from build123d import *

# Parameters (mm, degrees)
SKETCH1_R           = 16.995
SKETCH1_R_2         = 1.5
BOSS_EXTRUDE1_DEPTH = 5.08
CUT_EXTRUDE2_DEPTH  = 10


with BuildPart() as part:
    # Sketch1 → Boss-Extrude1 (new body)
    with BuildSketch(Plane.XY):
        Circle(SKETCH1_R)
        with Locations((-6.5, -11.258330249)):
            Circle(SKETCH1_R_2, mode=Mode.SUBTRACT)
        with Locations((6.5, -11.258330249)):
            Circle(SKETCH1_R_2, mode=Mode.SUBTRACT)
        with Locations((13, 0)):
            Circle(SKETCH1_R_2, mode=Mode.SUBTRACT)
        with Locations((6.5, 11.258330249)):
            Circle(SKETCH1_R_2, mode=Mode.SUBTRACT)
        with Locations((-6.5, 11.258330249)):
            Circle(SKETCH1_R_2, mode=Mode.SUBTRACT)
        with Locations((-13, 0)):
            Circle(SKETCH1_R_2, mode=Mode.SUBTRACT)
        with Locations((6.5, 11.258330249)):
            Circle(SKETCH1_R_2)
        with Locations((-6.5, -11.258330249)):
            Circle(SKETCH1_R_2)
    extrude(amount=BOSS_EXTRUDE1_DEPTH)

    # Sketch2 → Cut-Extrude2 (cut)
    with BuildSketch(Plane.XY.offset(5.08)):
        with BuildLine():
            ThreePointArc((-5.303300859, -8.131727984), (-5.303300859, -5.303300859), (-8.131727984, -5.303300859))
            Line((-8.131727984, -5.303300859), (-10.606601718, -7.778174593))
            ThreePointArc((-10.606601718, -7.778174593), (-10.606601718, -10.606601718), (-7.778174593, -10.606601718))
            Line((-7.778174593, -10.606601718), (-5.303300859, -8.131727984))
        make_face()
        with BuildLine():
            ThreePointArc((10.606601718, 7.778174593), (10.606601718, 10.606601718), (7.778174593, 10.606601718))
            Line((7.778174593, 10.606601718), (5.303300859, 8.131727984))
            ThreePointArc((5.303300859, 8.131727984), (5.303300859, 5.303300859), (8.131727984, 5.303300859))
            Line((8.131727984, 5.303300859), (10.606601718, 7.778174593))
        make_face()
    extrude(amount=-CUT_EXTRUDE2_DEPTH, mode=Mode.SUBTRACT)


solid = part.part
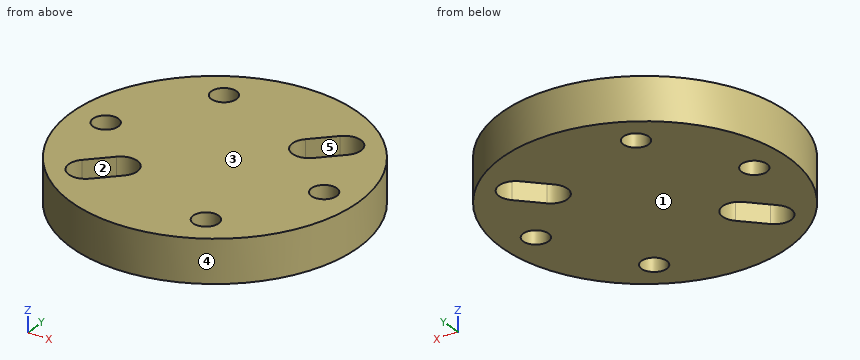
Source: CAD feature listing. Evaluate the final solid. Frame: model axes, mm. Face numbers are marked on the shaded views. A direction names the side the tool comes from. Coordinates: 2 decimals unless noted, no trailing zeros. Loops run counter-clockwise (first coordinate to the right, second up) from the corner with the lowest first, then second, coordinate; pieces in that order, holes last. Notation, with made-up numbers: (51, 15) -> (89, 15) arc R14 ccw to (89, 32) -> close; hole circle Ø9 at (-16.75, 87). An arc over 180 degrees is marked (long way). Answer in a Markdown table with one row per item. Add a question column.
Q1. Contact query for flat-ended pins moving along their axis: pin 1 Ø2 at (y, z) = (-8, 1.5) entering from +X; pin 2 Ø3 at (y, z) = (6, 3) entering from -X. Output: stop coordinate, or through.
Q2. Section C-C on x = -6.5. Return the cut outline in (y, z), and give its area (3 significant figures).
Q3. Section D-D on y = 12. Return the cut outline in (x, z), and give its area (3 significant figures).
Q4. Section A-A on y = 0. Return the cut outline in (x, z) (3 decimals), and give its area (3 significant figures).
Q5. Section B-B on x = 13. Return the cut outline in (y, z).
Q6. Pull-direction query (X, two-part tool) for the marked faces 3, 4 and 5; classes: pulls with the +X half, pulls with the -X half, needs draft (parallel to the pull), parting line crosses it, or undercut.
Q7. Reachability of the marked faces 1 and 2 from +Z, -Z, +X, -X, +Y, -Y: full face, straight path, thin tool, end or side. Return the list, or none.
Q8. Ray query, line 1 along X through (y, z) = (0.5, 4.35); line 2 along Y through (x, z) = (6.5, 3.8); line 3 along Y through (x, z) = (-7.5, 4.5). Return the intervals inside material, ascending.
Computed values:
| question | item | result |
|---|---|---|
| 1 | pin 1 | stops at x = 15.49 |
| 1 | pin 2 | stops at x = -16.39 |
| 2 | outline | (-15.7, 0) -> (-9.33, 0) -> (-9.33, 5.08) -> (-15.7, 5.08) -> close; (-4.73, 0) -> (9.76, 0) -> (9.76, 5.08) -> (-4.73, 5.08) -> close; (12.76, 0) -> (15.7, 0) -> (15.7, 5.08) -> (12.76, 5.08) -> close |
| 2 | area | 121 mm^2 |
| 3 | outline | (-12.03, 0) -> (-7.8, 0) -> (-7.8, 5.08) -> (-12.03, 5.08) -> close; (-5.2, 0) -> (12.03, 0) -> (12.03, 5.08) -> (-5.2, 5.08) -> close |
| 3 | area | 109 mm^2 |
| 4 | outline | (-16.995, 0) -> (-14.5, 0) -> (-14.5, 5.08) -> (-16.995, 5.08) -> close; (-11.5, 0) -> (11.5, 0) -> (11.5, 5.08) -> (-11.5, 5.08) -> close; (14.5, 0) -> (16.995, 0) -> (16.995, 5.08) -> (14.5, 5.08) -> close |
| 4 | area | 142 mm^2 |
| 5 | outline | (-10.95, 0) -> (-1.5, 0) -> (-1.5, 5.08) -> (-10.95, 5.08) -> close; (1.5, 0) -> (10.95, 0) -> (10.95, 5.08) -> (1.5, 5.08) -> close |
| 6 | face 3 | needs draft |
| 6 | face 4 | parting line crosses it |
| 6 | face 5 | undercut |
| 7 | face 1 | -Z, +X, -X, +Y, -Y |
| 7 | face 2 | +Z, -Z |
| 8 | line 1 | x = -16.99 to -14.41, -11.59 to 11.59, 14.41 to 16.99 |
| 8 | line 2 | y = -15.7 to -12.76, -9.76 to 4.73, 9.33 to 15.7 |
| 8 | line 3 | y = -15.25 to -10.33, -4.88 to 10.14, 12.38 to 15.25 |
